Part model, mm, in its own coordinate system. A direction names the side the tool comes from. Coordinates: 2 decimals unless noted, no trailing zeros. Order: outer loops, then holes, each group sorted by start corner. A loop starts at its lowest first (then second) coordinate and runs counter-clockwise, first axis right, second up.
from build123d import *

# Parameters (mm, degrees)
EXTRUDE_1_DEPTH     = 12.5
SKETCH_2_R          = 2.5
CUT_EXTRUDE_2_DEPTH = 52.53882032
CUT_EXTRUDE_3_REACH = 56.601
SKETCH_3_R          = 2


with BuildPart() as part:
    # Эскиз1 → Вытянуть1 (new body)
    with BuildSketch(Plane.XY):
        Polygon((0, 0), (0, 5), (10, 5), (10, 40), (15.9, 40), (15.9, 5), (24.1, 5), (24.1, 40), (30, 40), (30, 5), (40, 5), (40, 0), align=None)
    extrude(amount=EXTRUDE_1_DEPTH)

    # Эскиз2 → Вытянуть2 (cut, through all)
    with BuildSketch(Plane.ZY.offset(-10)):
        with Locations((6.25, 30)):
            Circle(SKETCH_2_R)
    extrude(amount=-CUT_EXTRUDE_2_DEPTH, mode=Mode.SUBTRACT)

    # Эскиз3 → Вытянуть3 (cut, up to next)
    with BuildSketch(Plane(origin=(0, 5, 0), x_dir=(1, 0, 0), z_dir=(0, 1, 0)), mode=Mode.PRIVATE) as cut_extrude_3_sk1:
        with Locations(Location((35, -6.25, 0), (0, 0, 270))):
            Circle(SKETCH_3_R)
    cut_extrude_3_tool1 = extrude(cut_extrude_3_sk1.sketch, amount=-CUT_EXTRUDE_3_REACH, mode=Mode.PRIVATE) & part.part
    # Эскиз3 → Вытянуть3 (cut, up to next)
    with BuildSketch(Plane(origin=(0, 5, 0), x_dir=(1, 0, 0), z_dir=(0, 1, 0)), mode=Mode.PRIVATE) as cut_extrude_3_sk2:
        with Locations(Location((5, -6.25, 0), (0, 0, 270))):
            Circle(SKETCH_3_R)
    cut_extrude_3_tool2 = extrude(cut_extrude_3_sk2.sketch, amount=-CUT_EXTRUDE_3_REACH, mode=Mode.PRIVATE) & part.part
    add(cut_extrude_3_tool1.solids().sort_by_distance((35, 5, 6.25))[0], mode=Mode.SUBTRACT)
    add(cut_extrude_3_tool2.solids().sort_by_distance((5, 5, 6.25))[0], mode=Mode.SUBTRACT)


solid = part.part
Q1. Cut at C-C on z = 6.25. Write the cut outline in (x, y).
Results list:
outline: (0, 0) - (3, 0) - (3, 5) - (0, 5) - close; (7, 0) - (33, 0) - (33, 5) - (30, 5) - (30, 27.5) - (24.1, 27.5) - (24.1, 5) - (15.9, 5) - (15.9, 27.5) - (10, 27.5) - (10, 5) - (7, 5) - close; (10, 32.5) - (15.9, 32.5) - (15.9, 40) - (10, 40) - close; (24.1, 32.5) - (30, 32.5) - (30, 40) - (24.1, 40) - close; (37, 0) - (40, 0) - (40, 5) - (37, 5) - close
Q2. Cut at D-D on z = 1.75. Write the cut outline in (x, y), and give its area (3 significant figures).
Results list:
outline: (0, 0) - (40, 0) - (40, 5) - (30, 5) - (30, 40) - (24.1, 40) - (24.1, 5) - (15.9, 5) - (15.9, 40) - (10, 40) - (10, 5) - (0, 5) - close
area: 613 mm2
Q3. Wall check: line 1 along X through (y, z) = (2.05, 6.25); line 2 along X through (y, z) = (18.5, 7.25); line 3 along Y through (x, z) = (28.5, 6.25). Give the ranges that are in metal, low to high.
Results list:
line 1: x = 0 to 3, 7 to 33, 37 to 40
line 2: x = 10 to 15.9, 24.1 to 30
line 3: y = 0 to 27.5, 32.5 to 40
Q4. Cut at A-A on x = 5. Write the cut outline in (y, z).
Results list:
outline: (0, 0) - (5, 0) - (5, 4.25) - (0, 4.25) - close; (0, 8.25) - (5, 8.25) - (5, 12.5) - (0, 12.5) - close
Q5. Cut at B-B on y = 13.5. Write the cut outline in (x, z).
Results list:
outline: (10, 0) - (15.9, 0) - (15.9, 12.5) - (10, 12.5) - close; (24.1, 0) - (30, 0) - (30, 12.5) - (24.1, 12.5) - close
Q6. Which spindle directions (+Z, -Z, +X, -X, +Y, -Y) get a long thin tool onto all of the face, cutting with end or side? Do faces 1 (the face through (24.1, 22, 6)), 2 (the face through (37.2, 5, 6.2)), 3 (the face through (7.2, 5, 6.2)). Say none if no direction does.
Results list:
face 1: +Z, -Z, +Y
face 2: +Z, -Z, +X, +Y
face 3: +Z, -Z, -X, +Y
Q7. Mould opens along Z. For faces 4 (the face through (25, 20, 0)), 5 (the face through (30, 23, 6)), 6 (the face through (12.91, 32.11, 7.59)) say: pulls with the +Z half, pulls with the -Z half, needs draft (parallel to the pull), parting line crosses it, or undercut.
Results list:
face 4: pulls with the -Z half
face 5: needs draft
face 6: undercut
Q8. Pin check, flat tips, straight feed: pin 1 Ø4 at (y, z) = (30, 6.25) entering from +X; pin 2 Ø2 at (y, z) = (26, 10) entering from -X; pin 3 Ø5 at (x, z) = (35, 6.25) entering from +Y; pin 4 Ø6 at (y, z) = (30.5, 6.5) entering from +X. Stop position of each tip, or through.
Results list:
pin 1: passes through
pin 2: stops at x = 10
pin 3: stops at y = 5
pin 4: stops at x = 30
